Could you check a few things on this model? Use its own coordinates, in mm. Face numbers are marked on the shaded views. A direction names the side the tool comes from. Coordinates: 2 decimals unless noted, no trailing zeros. Loops run counter-clockwise (first coordinate to the right, second up) from the corner with the lowest first, then second, coordinate; pieces in that order, holes last. Notation, with made-up numbers: (-16, 15) - (2, 15) arc R21 ccw to (2, 37) - close; hole circle Ø8 at (77.25, 49.5). An arc over 180 degrees is marked (long way). One line per question, with ' | ' between items. Start each with the question number.
1. Which directions (+Z, -Z, +X, -X, +Y, -Y) give clear straight access to the entire face, cutting with the end or side of a thin tool? Please do the marked faces 1, 2, 3 and 4.
2. I want a section at C-C, the plane y = 6.25. Count the separate pieces of the cut face and the enclosed holes in it, then the cut area to 3 significant figures.
3. We'd pull the mould along X, two halves only. Please class the marked faces 5, 6 and 7: pulls with the +X half, pulls with the -X half, needs draft (parallel to the pull), parting line crosses it, or undercut.
4. I want a section at D-D, the plane x = 48. Write out the boundary of the cut face in (y, z), then the cut area to 3 significant figures.
5. I want a section at B-B, the plane z = 6. Write out the boundary of the cut face in (x, y), then the cut area to 3 significant figures.
6. Please list where these lines run through material, in increasing order: L1, parallel to Y at x = 23, z = 2.5; L2, parallel to X at y = 16, z = 5.75; L3, parallel to Y at x = 27.5, z = 2.5. Write a range as [from, to].
7. I want a section at A-A, the plane x = 17. Write out the boundary of the cut face in (y, z), then the cut area to 3 significant figures.
8. I'm going to push flat-ended pins straight in: P1, Ø1.4, axis at x = 16, z = 6, coming from the -Y side; P2, Ø0.9, axis at x = 42.5, z = 3.5, coming from the -Y side; P3, Ø2, axis at x = 29, z = 6, coming from the +Y side. Where does each tip first touch, or does it pass through?
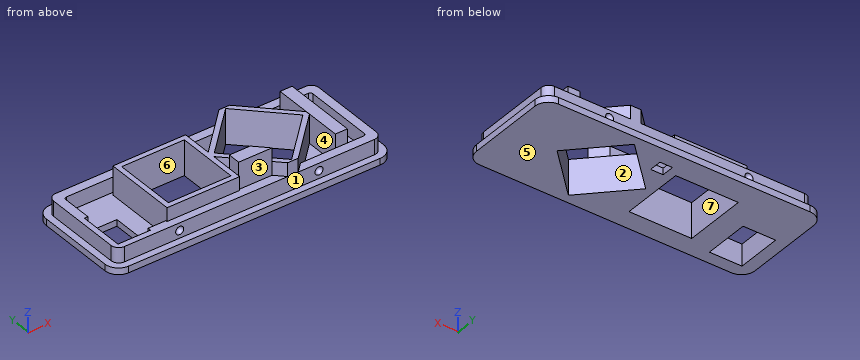
from build123d import *

# Parameters (mm, degrees)
BOSS_EXTRUDE1_DEPTH = 1.3
BOSS_EXTRUDE3_DEPTH = 3
CUT_EXTRUDE1_DEPTH  = 3
SKETCH11_W          = 6.5
SKETCH11_H          = 9
CUT_EXTRUDE2_DEPTH  = 4.3
SKETCH12_W          = 12.5
SKETCH12_H          = 12.5
CUT_EXTRUDE4_DEPTH  = 1.3
SKETCH17_W          = 14.5
SKETCH17_H          = 14.5
SKETCH17_W_2        = 12.5
SKETCH17_H_2        = 12.5
BOSS_EXTRUDE4_DEPTH = 7
CUT_EXTRUDE5_DEPTH  = 4.3
BOSS_EXTRUDE5_DEPTH = 7
CUT_EXTRUDE6_START  = -3
CUT_EXTRUDE6_DEPTH  = 23
SKETCH21_W          = 2.5
SKETCH21_H          = 2.5
CUT_EXTRUDE7_DEPTH  = 10
SKETCH23_W          = 2.4
SKETCH23_H          = 14.8
BOSS_EXTRUDE6_DEPTH = 5.75
BOSS_EXTRUDE7_DEPTH = 8.35


with BuildPart() as part:
    # Sketch1 → Boss-Extrude1 (new body)
    with BuildSketch(Plane.XY):
        with BuildLine():
            Line((2.7, 0), (52.9, 0))
            ThreePointArc((52.9, 0), (54.809188309, 0.790811691), (55.6, 2.7))
            Line((55.6, 2.7), (55.6, 18.4))
            ThreePointArc((55.6, 18.4), (54.809188309, 20.309188309), (52.9, 21.1))
            Line((52.9, 21.1), (2.7, 21.1))
            ThreePointArc((2.7, 21.1), (0.790811691, 20.309188309), (0, 18.4))
            Line((0, 18.4), (0, 2.7))
            ThreePointArc((0, 2.7), (0.790811691, 0.790811691), (2.7, 0))
        make_face()
    extrude(amount=BOSS_EXTRUDE1_DEPTH)

    # Sketch4 → Boss-Extrude3 (add)
    with BuildSketch(Plane.XY.offset(1.3)):
        with BuildLine():
            Line((54.25, 2.85), (54.25, 18.25))
            ThreePointArc((54.25, 18.25), (53.810660172, 19.310660172), (52.75, 19.75))
            Line((52.75, 19.75), (2.85, 19.75))
            ThreePointArc((2.85, 19.75), (1.789339828, 19.310660172), (1.35, 18.25))
            Line((1.35, 18.25), (1.35, 2.85))
            ThreePointArc((1.35, 2.85), (1.789339828, 1.789339828), (2.85, 1.35))
            Line((2.85, 1.35), (52.75, 1.35))
            ThreePointArc((52.75, 1.35), (53.810660172, 1.789339828), (54.25, 2.85))
        make_face()
    extrude(amount=BOSS_EXTRUDE3_DEPTH)

    # Sketch5 → Cut-Extrude1 (cut)
    with BuildSketch(Plane.XY.offset(4.3)):
        with BuildLine():
            Line((51.95, 17.95), (3.65, 17.95))
            ThreePointArc((3.65, 17.95), (3.296446609, 17.803553391), (3.15, 17.45))
            Line((3.15, 17.45), (3.15, 3.65))
            ThreePointArc((3.15, 3.65), (3.296446609, 3.296446609), (3.65, 3.15))
            Line((3.65, 3.15), (51.95, 3.15))
            ThreePointArc((51.95, 3.15), (52.303553391, 3.296446609), (52.45, 3.65))
            Line((52.45, 3.65), (52.45, 17.45))
            ThreePointArc((52.45, 17.45), (52.303553391, 17.803553391), (51.95, 17.95))
        make_face()
    extrude(amount=-CUT_EXTRUDE1_DEPTH, mode=Mode.SUBTRACT)

    # Sketch10 → Cut-Revolve1 (revolve, cut)
    with BuildSketch(Plane(origin=(0, 19.75, 0), x_dir=(1, 0, 0), z_dir=(0, 1, 0))):
        with BuildLine():
            Line((41.7, -2), (41.7, -3.6))
            ThreePointArc((41.7, -3.6), (40.9, -2.8), (41.7, -2))
        make_face()
    cut_revolve1 = revolve(axis=Axis((41.7, 19.75, 2), (0, 0, 1)), mode=Mode.SUBTRACT)

    # Mirror1: Cut-Revolve1 across plane
    add(cut_revolve1.mirror(Plane(origin=(0, 10.55, 0), x_dir=(0, 0, 1), z_dir=(0, -1, 0))), mode=Mode.SUBTRACT)

    # Sketch11 → Cut-Extrude2 (cut)
    with BuildSketch(Plane(origin=(0, 0, 0), x_dir=(-1, 0, 0), z_dir=(0, 0, -1))):
        with Locations((-5.7, 7)):
            Rectangle(SKETCH11_W, SKETCH11_H)
    extrude(amount=-CUT_EXTRUDE2_DEPTH, mode=Mode.SUBTRACT)

    # Sketch12 → Cut-Extrude4 (cut)
    with BuildSketch(Plane(origin=(0, 0, 0), x_dir=(-1, 0, 0), z_dir=(0, 0, -1))):
        with Locations((-19.75, 10.1)):
            Rectangle(SKETCH12_W, SKETCH12_H)
    extrude(amount=-CUT_EXTRUDE4_DEPTH, mode=Mode.SUBTRACT)

    # Sketch17 → Boss-Extrude4 (add)
    with BuildSketch(Plane(origin=(0, 0, 0), x_dir=(-1, 0, 0), z_dir=(0, 0, -1))):
        with Locations((-19.75, 10.1)):
            Rectangle(SKETCH17_W, SKETCH17_H)
        with Locations((-19.75, 10.1)):
            Rectangle(SKETCH17_W_2, SKETCH17_H_2, mode=Mode.SUBTRACT)
    extrude(amount=-BOSS_EXTRUDE4_DEPTH)

    # Sketch13 → Cut-Extrude5 (cut)
    with BuildSketch(Plane(origin=(0, 0, 0), x_dir=(-1, 0, 0), z_dir=(0, 0, -1))):
        Polygon((-45.338834765, 10.55), (-36.5, 1.711165235), (-27.661165235, 10.55), (-36.5, 19.388834765), align=None)
    extrude(amount=-CUT_EXTRUDE5_DEPTH, mode=Mode.SUBTRACT)

    # Sketch18 → Boss-Extrude5 (add)
    with BuildSketch(Plane(origin=(0, 0, 0), x_dir=(-1, 0, 0), z_dir=(0, 0, -1))):
        Polygon((-46.753048327, 10.55), (-36.5, 0.296951673), (-26.246951673, 10.55), (-36.5, 20.803048327), align=None)
        Polygon((-36.5, 19.388834765), (-45.338834765, 10.55), (-36.5, 1.711165235), (-27.661165235, 10.55), align=None, mode=Mode.SUBTRACT)
    extrude(amount=-BOSS_EXTRUDE5_DEPTH)

    # Sketch20 → Cut-Extrude6 (cut)
    with BuildSketch(Plane.XY.offset(4.3).offset(CUT_EXTRUDE6_START)):
        Polygon((35.446951673, 19.75), (37.553048327, 19.75), (36.5, 20.803048327), align=None)
    cut_extrude6 = extrude(amount=CUT_EXTRUDE6_DEPTH, mode=Mode.SUBTRACT)

    # Mirror2: Cut-Extrude6 across plane
    add(cut_extrude6.mirror(Plane(origin=(0, 10.55, 0), x_dir=(0, 0, 1), z_dir=(0, -1, 0))), mode=Mode.SUBTRACT)

    # Sketch21 → Cut-Extrude7 (cut)
    with BuildSketch(Plane(origin=(0, 0, 0), x_dir=(-1, 0, 0), z_dir=(0, 0, -1))):
        with Locations((-29, 16.6)):
            Rectangle(SKETCH21_W, SKETCH21_H)
    extrude(amount=-CUT_EXTRUDE7_DEPTH, mode=Mode.SUBTRACT)

    # Mirror3: Cut-Revolve1 across plane
    add(cut_revolve1.mirror(Plane.ZY.offset(-27.8)), mode=Mode.SUBTRACT)

    # Mirror3 copy 1 sketch → Mirror3 copy 1 (revolve, cut)
    with BuildSketch(Plane(origin=(55.6, 1.35, 0), x_dir=(-1, 0, 0), z_dir=(0, -1, 0))):
        with BuildLine():
            Line((41.7, -2), (41.7, -3.6))
            ThreePointArc((41.7, -3.6), (40.9, -2.8), (41.7, -2))
        make_face()
    revolve(axis=Axis((13.9, 1.35, 2), (0, 0, 1)), mode=Mode.SUBTRACT)

    # Sketch23 → Boss-Extrude6 (add)
    with BuildSketch(Plane.XY.offset(1.3)):
        with Locations((47.5, 10.55)):
            Rectangle(SKETCH23_W, SKETCH23_H)
    extrude(amount=BOSS_EXTRUDE6_DEPTH)

    # Sketch24 → Boss-Extrude7 (add)
    with BuildSketch(Plane.XY.offset(1.3)):
        Polygon((33.646951673, 3.15), (27, 3.15), (27, 5.65), (31.146951673, 5.65), align=None)
    extrude(amount=BOSS_EXTRUDE7_DEPTH)


solid = part.part
Results are:
1) face 1: +Z, +X, -X, -Y | face 2: +Z, -Z | face 3: +Z, -Y | face 4: +Z
2) separate pieces: 4 | enclosed holes: 0 | area: 85.8 mm2
3) face 5: needs draft | face 6: undercut | face 7: undercut
4) outline: (0, 0) - (21.1, 0) - (21.1, 1.3) - (19.75, 1.3) - (19.75, 4.3) - (17.95, 4.3) - (17.95, 7.05) - (3.15, 7.05) - (3.15, 4.3) - (1.35, 4.3) - (1.35, 1.3) - (0, 1.3) - close | area: 123 mm2
5) outline: (12.5, 2.85) - (27, 2.85) - (27, 3.15) - (33.65, 3.15) - (35.45, 1.35) - (37.55, 1.35) - (46.3, 10.1) - (46.3, 3.15) - (48.7, 3.15) - (48.7, 17.95) - (46.3, 17.95) - (46.3, 11) - (37.55, 19.75) - (35.45, 19.75) - (27, 11.3) - (27, 17.35) - (12.5, 17.35) - close; hole (13.5, 3.85) - (26, 3.85) - (26, 16.35) - (13.5, 16.35) - close; hole (27, 5.65) - (31.15, 5.65) - (27, 9.8) - close; hole (27.66, 10.55) - (36.5, 1.71) - (45.34, 10.55) - (36.5, 19.39) - close | area: 154 mm2
6) L1: y = [1.35, 3.85], [16.35, 17.35], [17.95, 19.75] | L2: x = [12.5, 13.5], [26, 27], [31.7, 33.11], [39.89, 41.3], [46.3, 48.7] | L3: y = [1.35, 5.65], [9.3, 11.8], [17.95, 19.75]
7) outline: (0, 0) - (3.85, 0) - (3.85, 7) - (2.85, 7) - (2.85, 4.3) - (1.35, 4.3) - (1.35, 1.3) - (0, 1.3) - close; (16.35, 0) - (21.1, 0) - (21.1, 1.3) - (19.75, 1.3) - (19.75, 4.3) - (17.95, 4.3) - (17.95, 1.3) - (17.35, 1.3) - (17.35, 7) - (16.35, 7) - close | area: 32.5 mm2
8) P1: stops at y = 2.85 | P2: stops at y = 1.35 | P3: stops at y = 14.3
